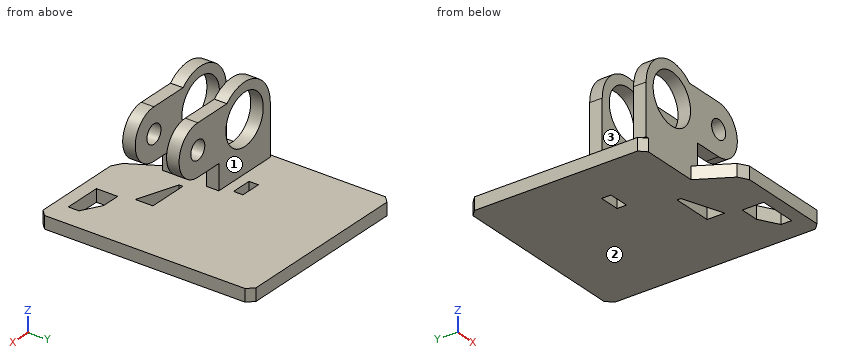
```python
from build123d import *

# Parameters (mm, degrees)
SKETCH2_W           = 33
SKETCH2_H           = 15
BOSS_EXTRUDE1_DEPTH = 20
SKETCH7_R           = 40
SKETCH7_R_2         = 15
BOSS_EXTRUDE5_DEPTH = 20
LPATTERN2_COUNT     = 2
LPATTERN2_PITCH     = 70


with BuildPart() as part:
    # Sketch2 → Boss-Extrude1 (new body)
    with BuildSketch(Plane.XY):
        Polygon((-140, -110), (-48.782097787, -110), (-19.141081636, -161.339745962), (-4.141081636, -170), (140, -170), (150, -160), (150, 160), (140, 170), (-140, 170), (-150, 160), (-150, -100), align=None)
        Polygon((84, -115), (114, -132), (114, -149), (54, -149), (54, -115), align=None, mode=Mode.SUBTRACT)
        Polygon((47, -92), (-17, -70), (-17, -64), (47, -64), align=None, mode=Mode.SUBTRACT)
        with Locations((-61.5, 3.5)):
            Rectangle(SKETCH2_W, SKETCH2_H, mode=Mode.SUBTRACT)
    extrude(amount=BOSS_EXTRUDE1_DEPTH)

    # Sketch7 → Boss-Extrude5 (add)
    with BuildSketch(Plane.XZ.offset(110)):
        with BuildLine():
            Line((-145, 20), (-145, 100))
            ThreePointArc((-145, 100), (-111.780674121, 150.503487353), (-52.250827824, 140))
            Line((-52.250827824, 140), (10, 140))
            ThreePointArc((10, 140), (50, 100), (10, 60))
            Line((10, 60), (-35, 60))
            Line((-35, 60), (-35, 20))
            Line((-35, 20), (-145, 20))
        make_face()
        with Locations((-90, 100)):
            Circle(SKETCH7_R, mode=Mode.SUBTRACT)
        with Locations((10, 100)):
            Circle(SKETCH7_R_2, mode=Mode.SUBTRACT)
    boss_extrude5 = extrude(amount=-BOSS_EXTRUDE5_DEPTH)

    # LPattern2: Boss-Extrude5 ×2
    with Locations(*[(0, i * LPATTERN2_PITCH, 0) for i in range(1, LPATTERN2_COUNT)]):
        add(boss_extrude5)


solid = part.part
```
The listing builds one solid part. Answer for the finished solid, in the listing's coordinates (mm). Face numbers are marked on the shaded views. Coordinates: 2 decimals unless noted, no trailing zeros. Write each loop counter-clockwise with the first axis right and the second up, starting at its lowest first coordinate (ties: lowest second). Pieces come first, ordered by that corner, then holes.
Q1. Section A-A, the plane x = 93 is taken. Write down the section's boundary in (y, z).
Returned:
outline: (-170, 0) - (-149, 0) - (-149, 20) - (-170, 20) - close; (-120.1, 0) - (170, 0) - (170, 20) - (-120.1, 20) - close
Q2. Section C-C, the plane x = -10.5 is taken. Write down the section's boundary in (y, z), then the cut area to 3 significant figures.
Returned:
outline: (-166.33, 0) - (-72.23, 0) - (-72.23, 20) - (-166.33, 20) - close; (-110, 60) - (-90, 60) - (-90, 140) - (-110, 140) - close; (-64, 0) - (170, 0) - (170, 20) - (-64, 20) - close; (-40, 60) - (-20, 60) - (-20, 140) - (-40, 140) - close
area: 9,760 mm2
Q3. Section D-D, the plane x = -90 is taken. Write down the section's boundary in (y, z).
Returned:
outline: (-110, 0) - (170, 0) - (170, 20) - (-20, 20) - (-20, 60) - (-40, 60) - (-40, 20) - (-90, 20) - (-90, 60) - (-110, 60) - close; (-110, 140) - (-90, 140) - (-90, 155) - (-110, 155) - close; (-40, 140) - (-20, 140) - (-20, 155) - (-40, 155) - close
Q4. The mould has two halves that part along Y. Classify the marked faces 1, 2 and 3: released by +Y, released by -Y, zero draft, split by the parting line, or undercut.
Returned:
face 1: released by +Y
face 2: zero draft
face 3: undercut
Q5. Given P1, Ø3, axis at x = 2.5, y = 53, coming from the +Z side; P2, Ø10, axis at y = -28, z = 64.5, coming from the -X side; P3, Ø10, axis at y = -102, z = 43.5, coming from the +X side; P4, Ø24, axis at x = 10, z = 100, coming from the -Y side, each flat-ended and moving along its own axis, determine where each tip first touches the part or whether it passes through.
Returned:
P1: stops at z = 20
P2: stops at x = -145
P3: stops at x = -35
P4: passes through
Q6. Find the intervals of material crossed by line 1 along Z through (x, y) = (-90, -101); line 2 along Y through (x, z) = (-43, 134); line 3 along Z through (x, y) = (-103.5, 83), in increasing order.
Returned:
line 1: z = 0 to 60, 140 to 155
line 2: y = -110 to -90, -40 to -20
line 3: z = 0 to 20
Q7. Section B-B, the plane z = 90 is taken. Write down the section's boundary in (x, y), then the cut area to 3 significant figures.
Returned:
outline: (-145, -110) - (-128.73, -110) - (-128.73, -90) - (-145, -90) - close; (-145, -40) - (-128.73, -40) - (-128.73, -20) - (-145, -20) - close; (-51.27, -110) - (-1.18, -110) - (-1.18, -90) - (-51.27, -90) - close; (-51.27, -40) - (-1.18, -40) - (-1.18, -20) - (-51.27, -20) - close; (21.18, -110) - (48.73, -110) - (48.73, -90) - (21.18, -90) - close; (21.18, -40) - (48.73, -40) - (48.73, -20) - (21.18, -20) - close
area: 3,760 mm2
